from build123d import *

# Parameters (mm, degrees)
BOSS_EXTRUDE1_DEPTH = 50
BOSS_EXTRUDE2_DEPTH = 2.5
BOSS_EXTRUDE3_DEPTH = 1
SKETCH4_W           = 1
SKETCH4_H           = 5
BOSS_EXTRUDE4_DEPTH = 3


with BuildPart() as part:
    # Sketch1 → Boss-Extrude1 (new body)
    with BuildSketch(Plane.XY):
        with BuildLine():
            Line((21.476731595, 1), (24.47958333, 1))
            ThreePointArc((24.47958333, 1), (-24.5, 0), (24.47958333, -1))
            Line((24.47958333, -1), (21.476731595, -1))
            ThreePointArc((21.476731595, -1), (-21.5, 0), (21.476731595, 1))
        make_face()
    extrude(amount=BOSS_EXTRUDE1_DEPTH)

    # Sketch2 → Boss-Extrude2 (add, symmetric)
    with BuildSketch(Plane.XY.offset(25)):
        with BuildLine():
            Line((24.47958333, 1), (29.171263931, 1))
            Line((29.171263931, 1), (29.171263931, 4))
            Line((29.171263931, 4), (24.171263931, 4))
            ThreePointArc((24.171263931, 4), (24.37162766, 2.504748533), (24.47958333, 1))
        make_face()
        with BuildLine():
            Line((29.171263931, -4), (24.171263931, -4))
            ThreePointArc((24.171263931, -4), (24.37162766, -2.504748533), (24.47958333, -1))
            Line((24.47958333, -1), (29.171263931, -1))
            Line((29.171263931, -1), (29.171263931, -4))
        make_face()
    extrude(amount=BOSS_EXTRUDE2_DEPTH, both=True)

    # Sketch3 → Boss-Extrude3 (add, symmetric)
    with BuildSketch(Plane.XY.offset(25)):
        with BuildLine():
            Line((20.976176963, 1), (21.476731595, 1))
            ThreePointArc((21.476731595, 1), (-21.5, 0), (21.476731595, -1))
            Line((21.476731595, -1), (20.976176963, -1))
            ThreePointArc((20.976176963, -1), (-21, 0), (20.976176963, 1))
        make_face()
    extrude(amount=BOSS_EXTRUDE3_DEPTH, both=True)

    # Sketch4 → Boss-Extrude4 (add)
    with BuildSketch(Plane(origin=(0, 4, 0), x_dir=(1, 0, 0), z_dir=(0, 1, 0))):
        with Locations((28.671263931, -25)):
            Rectangle(SKETCH4_W, SKETCH4_H)
    boss_extrude4 = extrude(amount=BOSS_EXTRUDE4_DEPTH)

    # Mirror1: Boss-Extrude4 across plane
    add(boss_extrude4.mirror(Plane.ZX))


solid = part.part
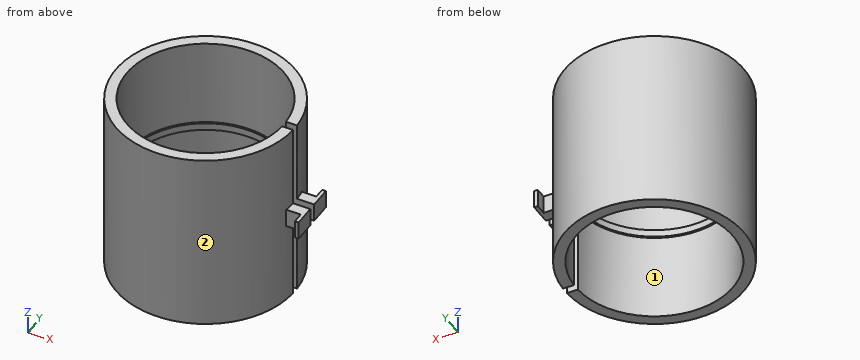
Model file for the job. Use its own axes, mm. Face numbers are marked on the shaded views. Give positions to 0.01 mm unless a question says otherwise; leave off trailing zeros. Order: outer loops, then holes, each group sorted by start corner. A loop starts at its lowest first (then second) coordinate and runs counter-clockwise, first axis right, second up. Notation, with made-up numbers: M -33.75,36.5 L 18.25,36.5 A14 cw 18.25,47.5 Z; hole C -0.75,-34 d9. An arc over 180 degrees is marked long. Write item = value, one per line.
Q1. Cut at B-B, the plane y = 0. List the corners of the cut face in (x, z), then the cut area to 3 significant figures.
Derived:
outline = M -24.5,0 L -21.5,0 L -21.5,24 L -21,24 L -21,26 L -21.5,26 L -21.5,50 L -24.5,50 Z
area = 151 mm2
Q2. Two-plate mould, pull along Y, no slides. Class the marked faces 1 and 2: pulls with the +Y half, pulls with the -Y half, needs draft (parallel to the pull), parting line crosses it, or undercut.
Derived:
face_1 = undercut
face_2 = parting line crosses it
Q3. Flat gauge pins, fed straight in: pin 1 (6 mm diameter, centred on x = -12, z = 6, fed in from +Y); pin 2 (4.5 mm diameter, centred on x = 26, z = 24, fed in from -Y); pin 3 (1 mm diameter, centred on x = 12.5, z = 28.5, fed in from -Y). Where does each tip first touch, or does it go through?
Derived:
pin_1 = 22.79
pin_2 = -7
pin_3 = -21.36
Q4. Drill centre lines: line 1 (X direction, y = 15.5, z = 22); line 2 (Y direction, x = 0, z = 25.15); line 3 (X direction, y = 13.5, z = 24.5). Where is each one in solid material? Low to high. Write a range as [from, to].
Derived:
line_1 = [-18.97, -14.9], [14.9, 18.97]
line_2 = [-24.5, -21], [21, 24.5]
line_3 = [-20.45, -16.09], [16.09, 20.45]
Q5. Cut at D-D, the plane y = 19.5. List the corners of the cut face in (x, z).
Derived:
outline = M -14.83,0 L -9.06,0 L -9.06,24 L -7.79,24 L -7.79,26 L -9.06,26 L -9.06,50 L -14.83,50 Z; M 7.79,24 L 9.06,24 L 9.06,0 L 14.83,0 L 14.83,50 L 9.06,50 L 9.06,26 L 7.79,26 Z
Q6. Cut at A-A, the plane x = 26.5. List the corners of the cut face in (y, z).
Derived:
outline = M -4,22.5 L -1,22.5 L -1,27.5 L -4,27.5 Z; M 1,22.5 L 4,22.5 L 4,27.5 L 1,27.5 Z
Q7. Cut at C-C, the plane x = 0. List the corners of the cut face in (y, z), then the cut area to 3 significant figures.
Derived:
outline = M -24.5,0 L -21.5,0 L -21.5,24 L -21,24 L -21,26 L -21.5,26 L -21.5,50 L -24.5,50 Z; M 21,24 L 21.5,24 L 21.5,0 L 24.5,0 L 24.5,50 L 21.5,50 L 21.5,26 L 21,26 Z
area = 302 mm2
